Can you work these out from the model? Positions are in its coordinate system, mm. A direction names the side the tool comes from. Round coordinates to 2 decimals unless told otherwise and drop trailing zeros. Loops run counter-clockwise (first coordinate to the right, second up) from the corner with the lowest first, then second, coordinate; pieces in that order, holes last. Notation, with made-up numbers: (31, -13) - (63, -13) arc R12 cw to (63, 2) - close; hole circle Ø8 at (30.25, -23). An arc over 180 degrees is marked (long way). Answer as CSV lines item,"result".
Autodesk Inventor part; units mm, degrees
ref_plane "YZ Plane" through (0, 0, 0) normal (1, 0, 0) x (0, 1, 0)
ref_plane "XZ Plane" through (0, 0, 0) normal (0, 1, 0) x (-1, 0, 0)
ref_plane "XY Plane" through (0, 0, 0) normal (0, 0, 1) x (1, 0, 0)
sketch "Sketch1" plane through (0, 0, 0) normal (0, 0, 1) x (1, 0, 0)
  line L0 (14.1, 28.2) -> (14.1, 0)
  line L1 (14.1, 0) -> (-14.1, 0)
  line L2 (-14.1, 0) -> (-14.1, 4)
  line L3 (-14.1, 4) -> (10.1, 4)
  line L4 (10.1, 4) -> (10.1, 28.2)
  line L5 (10.1, 28.2) -> (14.1, 28.2)
  point P0 (0, 0)
  point P1 (0, 0)
  dimension "d0" = 28.2
  dimension "d1" = 4
extrude "Escuadra cuerpo" add sketch "Sketch1" along normal mid plane 20
sketch "Sketch2" plane through (0, 0, 10) normal (0, 0, 1) x (1, 0, 0)
  line L0 (10.1, 4) -> (-14.1, 4)
  line L1 (-9.1, 4) -> (10.1, 23.2)
  line L2 (10.1, 23.2) -> (10.1, 4)
  line L3 (10.1, 4) -> (-9.1, 4)
  line L4 (14.1, 28.2) -> (10.1, 28.2)
  point P0 (0, 0)
  dimension "d4" = 5
  dimension "d5" = 5
extrude "Nervia lateral 1" add sketch "Sketch2" against normal blind 2.5
sketch "Sketch3" plane through (0, 0, -10) normal (0, 0, -1) x (-1, 0, 0)
  line L0 (-10.1, 4) -> (-10.1, 23.2)
  line L1 (-10.1, 23.2) -> (9.1, 4)
  line L2 (14.1, 4) -> (-10.1, 4)
  line L3 (-10.1, 4) -> (-10.1, 28.2)
  line L4 (-10.1, 23.2) -> (-10.1, 4)
  line L5 (-10.1, 4) -> (9.1, 4)
  point P0 (0, 0)
  dimension "d8" = 5
  dimension "d9" = 5
extrude "Nervio lateral 2" add sketch "Sketch3" against normal blind 2.5
sketch "Sketch4" plane through (-14.1, 0, 10) normal (0, -1, 0) x (1, 0, 0)
  point P0 (14.1, -10)
  point P1 (14.1, -10)
hole "BCC M6 1" at (0, 0, 0) direction (0, 1, 0) diameter 6.4 end through all
sketch "Sketch5" plane through (14.1, 0, 10) normal (1, 0, 0) x (0, 0, -1)
  line L0 (0, 0) -> (0, 28.2)
  line L1 (20, 0) -> (0, 0)
  point P0 (10, 0)
  point P1 (10, 14.1)
  point P2 (0, 14.1)
  point P3 (10, 0)
hole "BCC M5 2" at (14.1, 14.1, 0) direction (-1, 0, 0) diameter 6.4 end through all
properties part number "Escuadra DC"
Q1. Imagine slicing it at A-A (y = 14.1). Write out the boundary of the cut face in (x, z), then the cut area to 3 significant figures.
Checks:
outline,"(1, -10) - (14.1, -10) - (14.1, -3.2) - (10.1, -3.2) - (10.1, -7.5) - (1, -7.5) - close; (1, 7.5) - (10.1, 7.5) - (10.1, 3.2) - (14.1, 3.2) - (14.1, 10) - (1, 10) - close"
area,"99.9 mm²"
Q2. On a 3-axis mill with a long thin cutter (end or side, diameter ignored), from which of +Z, -Z, +X, -X, +Y, -Y can I reach the whole of each face in a straight line? I mean faces 1 (the flat face through (5, 9, 7.5)), 2 (the flat face through (6, 8, -10)). Say none if no direction works.
Checks:
face 1,"-X, +Y"
face 2,"-Z, +X, -X, +Y, -Y"
Q3. I'm going to push flat-ended pins straight in: pin 1 Ø1.5 at (y, z) = (12, -6) entering from -X; pin 2 Ø5 at (x, z) = (7.5, -0.5) entering from +Y; pin 3 Ø5 at (x, z) = (3, 8) entering from +Y. Where does each tip first touch, or does it pass through?
Checks:
pin 1,"x = 10.1"
pin 2,"y = 4"
pin 3,"y = 18.6"
Q4. Imagine slicing it at C-C (x = 4). Write out the boundary of the cut face in (y, z).
Checks:
outline,"(0, -10) - (17.1, -10) - (17.1, -7.5) - (4, -7.5) - (4, 7.5) - (17.1, 7.5) - (17.1, 10) - (0, 10) - close"
Q5. Imagine slicing it at B-B (x = 0). Write out the boundary of the cut face in (y, z).
Checks:
outline,"(0, -10) - (13.1, -10) - (13.1, -7.5) - (4, -7.5) - (4, -3.2) - (0, -3.2) - close; (0, 3.2) - (4, 3.2) - (4, 7.5) - (13.1, 7.5) - (13.1, 10) - (0, 10) - close"
Q6. Imagine slicing it at D-D (y = 2). Write out the boundary of the cut face in (x, z).
Checks:
outline,"(-14.1, -10) - (14.1, -10) - (14.1, 10) - (-14.1, 10) - close; hole circle Ø6.4 at (0, 0)"
Q7. We'd pull the mould along Z, two halves only. Please class faces 3 (the cylindrical face through (1.947, 2.028, 2.539)), 4 (the flat face through (3, 0, 2)), 5 (the flat face through (6, 8, 10)): pulls with the +Z half, pulls with the -Z half, needs draft (parallel to the pull), parting line crosses it, or undercut.
Checks:
face 3,"undercut"
face 4,"needs draft"
face 5,"pulls with the +Z half"
Q8. If I drill on line 1 along Y through (x, z) = (11.95, 0); line 2 along Z through (x, y) = (9.75, 14.5); line 3 along Z through (x, y) = (0, 2.15), over which ranges is the centre line in solid material (lowest first)? Write a range as [from, to].
Checks:
line 1,"[0, 10.9], [17.3, 28.2]"
line 2,"[-10, -7.5], [7.5, 10]"
line 3,"[-10, -3.2], [3.2, 10]"
